from build123d import *

# Parameters (mm, degrees)
F0_R     = 9.525
F1_DEPTH = 19.05
F2_R     = 12.7
F3_DEPTH = 3.175
F4_R     = 12.7
F4_R_2   = 9.525
F5_DEPTH = 3.175
F6_R     = 1.5875
F7_DEPTH = 25.4


with BuildPart() as f1:
    # F0 (on Top) → F1 (new body)
    with BuildSketch(Plane.XY):
        Circle(F0_R)
    extrude(amount=F1_DEPTH)

    # F2 (on Top) → F3 (join)
    with BuildSketch(Plane.XY):
        Circle(F2_R)
    extrude(amount=-F3_DEPTH)

    # F4 (on face) → F5 (join)
    with BuildSketch(Plane.XY.offset(19.05)):
        Circle(F4_R)
        Circle(F4_R_2, mode=Mode.SUBTRACT)
        Circle(F4_R_2)
    extrude(amount=F5_DEPTH)

    # F6 (on Top) → F7 (cut, symmetric)
    with BuildSketch(Plane.XY):
        Circle(F6_R)
    extrude(amount=F7_DEPTH, both=True, mode=Mode.SUBTRACT)


solid = f1.part
Geometry: final body of the model. Coordinates: model frame, mm. A direction names the side the tool comes from. Give positions to 0.01 mm unless a question says otherwise; leave off trailing zeros. Write each loop counter-clockwise with the first axis right and the second up, starting at its lowest first coordinate (ties: lowest second). Pieces come first, ordered by that corner, then holes. Notation, with made-up numbers: (44, 88.25) -> (71, 88.25) arc R3 ccw to (71, 92.25) -> close; hole circle Ø2 at (31.25, 36.25). An arc over 180 degrees is marked (long way). Answer in a Markdown table with one row per item.
(1) Ray query, line 1 along Z through (x, y) = (-7.25, 6.5) (3 decimals); line 2 along X through (y, z) = (1.25, 7.5); line 3 along Y through (x, z) = (1, 4.5). Return the intervals inside material, ascending. Write a range as [from, to].
Answers below:
| item | result |
|---|---|
| line 1 | [-3.175, 0], [19.05, 22.225] |
| line 2 | [-9.44, -0.98], [0.98, 9.44] |
| line 3 | [-9.47, -1.23], [1.23, 9.47] |
(2) Section query B-B on y = 7.75. Return loops of the section in (x, z) (3 decimals), then the cut area to 3 significant figures.
Answers below:
| item | result |
|---|---|
| outline | (-10.061, -3.175) -> (10.061, -3.175) -> (10.061, 0) -> (5.537, 0) -> (5.537, 19.05) -> (10.061, 19.05) -> (10.061, 22.225) -> (-10.061, 22.225) -> (-10.061, 19.05) -> (-5.537, 19.05) -> (-5.537, 0) -> (-10.061, 0) -> close |
| area | 339 mm^2 |
(3) Pin query (flat end, axial travel): pin 1 (3 mm diameter, centred on x = -7, z = 12, fed in from -Y); pin 2 (2 mm diameter, centred on x = 8.5, z = 10, fed in from +Y); pin 3 (10 mm diameter, centred on y = -4.5, z = 15.5, fed in from -X). Return the tip coordinate at first contact, or that it passes through.
Answers below:
| item | result |
|---|---|
| pin 1 | y = -7.78 |
| pin 2 | y = 5.87 |
| pin 3 | x = -12.66 |
(4) Set-up query: faces 5 (the flat face through (5, 9, 19.05)), 6 (the cylindrical face through (-2.75, -12.4, -1.57)). Return all of +Z, -Z, +X, -X, +Y, -Y with unobstructed straight access to the full face (end or side cutting, diameter ignored); none if empty.
Answers below:
| item | result |
|---|---|
| face 5 | none |
| face 6 | +Z, -Z |
(5) Draft query along Z for faces 1 (the flat face through (3, 0, 22.225)), 2 (the flat face through (5, 9, 0)), 3 (the cylindrical face through (-7.559, -5.796, 9.392)), 4 (the flat face through (3, 0, -3.175)). Return one class per face: +Z half, -Z half, draft (parallel to the pull), parting line (faces both ways), or undercut.
Answers below:
| item | result |
|---|---|
| face 1 | +Z half |
| face 2 | undercut |
| face 3 | undercut |
| face 4 | -Z half |
(6) Section query D-D on x = 4.75. Return loops of the section in (y, z) (3 decimals), then the cut area to 3 significant figures.
Answers below:
| item | result |
|---|---|
| outline | (-11.778, -3.175) -> (11.778, -3.175) -> (11.778, 0) -> (8.256, 0) -> (8.256, 19.05) -> (11.778, 19.05) -> (11.778, 22.225) -> (-11.778, 22.225) -> (-11.778, 19.05) -> (-8.256, 19.05) -> (-8.256, 0) -> (-11.778, 0) -> close |
| area | 464 mm^2 |
